Here's how the part is built. I have some questions about the finished solid (model axes, mm). A direction names the side the tool comes from. Coordinates: 2 decimals unless noted, no trailing zeros. Write each loop counter-clockwise with the first axis right and the second up, starting at its lowest first coordinate (ties: lowest second). Pieces come first, ordered by that corner, then holes. Notation, with made-up numbers: (30.25, 77.25) -> (87.25, 77.25) arc R12 cw to (87.25, 95.25) -> close; hole circle Ø2 at (44, 85.5). An arc over 180 degrees is marked (long way). Use a Markdown table: item, result. Add a question column.
Item 1: Imagine slicing it at B-B, the plane y = -6. Write out the boundary of the cut face in (x, z).
Item 2: If we mould it in two halves opening along X, with no side actions, what happens to faces 1 (the cylindrical face through (29.9, -19.94, 3.46)), 2 (the conical face through (-38.037, -20.598, 4.386)), 3 (the cylindrical face through (38.3, 20.74, 2.28))? For each: pulls with the +X half, pulls with the -X half, needs draft (parallel to the pull), parting line crosses it, or undercut.
Item 3: Will these pins go through, and if not, where does the flat tip stop? pin 1 Ø1.6 at (x, y) = (34, -18.5) entering from -Z; pin 2 Ø2.5 at (x, y) = (-35.3, 17.8) entering from -Z; pin 3 Ø1.5 at (x, y) = (23.5, 7) entering from +Z.
Item 4: On a 3-axis mill with a long thin cutter (end or side, diameter ignored), from which of +Z, -Z, +X, -X, +Y, -Y can I reach the whole of each face in a straight line? I mean faces 4 (the flat face through (37.67, -19.194, 1.331)), 5 (the conical face through (-38.098, 20.537, 4.386)), 6 (the flat face through (38.3, 4, 3)). Say none if no direction works.
Item 5: Imagine slicing it at A-A, the plane x = 0. Write out the boundary of the cut face in (y, z).
Item 6: If I drill on line 1 along X through (y, z) = (-17.8, 3.2); line 2 along X through (y, z) = (17.8, 3.15); line 3 along X through (y, z) = (9, 3.5), over which ranges is the centre line in solid material (lowest first)? Write a range as from..to.
Autodesk Fusion 360 part; units mm, degrees
sketch "Sketch1" plane through (0, 0, 0) normal (0, 0, 1) x (1, 0, 0)
  line L0 (39.5, 22) -> (-39.5, 22)
  line L1 (-39.5, 22) -> (-39.5, -22)
  line L2 (-39.5, -22) -> (39.5, -22)
  line L3 (39.5, -22) -> (39.5, 22)
  line L4 (39.5, 22) -> (-39.5, -22) construction
  line L5 (-39.5, 22) -> (39.5, -22) construction
  dimension "d1" = 44
  dimension "d2" = 79
extrude "Extrude1" add sketch "Sketch1" along normal blind 4.5
sketch "Sketch2" plane through (0, 0, 4.5) normal (0, 0, 1) x (-1, 0, 0)
  line L0 (-39.5, 22) -> (-39.5, -22)
  line L1 (-39.5, -22) -> (39.5, -22)
  line L2 (39.5, -22) -> (39.5, 22)
  line L3 (39.5, 22) -> (-39.5, 22)
  line L4 (-38.3, 20.8) -> (-38.3, -20.8)
  line L5 (-38.3, -20.8) -> (38.3, -20.8)
  line L6 (38.3, -20.8) -> (38.3, 20.8)
  line L7 (38.3, 20.8) -> (-38.3, 20.8)
  dimension "d5" = -1.2
extrude "Extrude2" cut sketch "Sketch2" against normal blind 2.1 contours L4 L5 L6 L7
sketch "Sketch3" plane through (0, 0, 2.4) normal (0, 0, 1) x (-1, 0, 0)
  line L0 (38.3, 20.8) -> (-38.3, 20.8)
  line L1 (-38.3, 20.8) -> (-38.3, -20.8)
  line L2 (-38.3, -20.8) -> (38.3, -20.8)
  line L3 (38.3, -20.8) -> (38.3, 20.8)
  line L4 (-38.3, -20.8) -> (-38.3, 20.8)
  line L5 (-38.3, 20.8) -> (38.3, 20.8)
  line L6 (38.3, 20.8) -> (38.3, -20.8)
  line L7 (38.3, -20.8) -> (-38.3, -20.8)
  line L8 (-39.5, 22) -> (-39.5, -22)
  line L9 (-39.5, -22) -> (39.5, -22)
  line L10 (39.5, -22) -> (39.5, 22)
  line L11 (39.5, 22) -> (-39.5, 22)
  circle A0 centre (35.3, -17.8) radius 4.5
  circle A1 centre (-35.3, 17.8) radius 4.5
  circle A2 centre (35.3, 17.8) radius 4.5
  dimension "d8" = 9
  dimension "d9" = 3
  dimension "d10" = 3
  dimension "d11" = 9
  dimension "d12" = 9
  dimension "d13" = 3
  dimension "d14" = 3
  dimension "d15" = 3
  dimension "d16" = 3
extrude "Extrude3" add sketch "Sketch3" along normal blind 2.1 contours L2 L3 L6 L7 A0
extrude "Extrude4" add sketch "Sketch3" along normal blind 2.1 contours L0 L3 L5 L6 A2
extrude "Extrude5" add sketch "Sketch3" along normal blind 2.1 contours L0 L1 L4 L5 A1
sketch "Sketch5" plane through (0, 0, 4.5) normal (0, 0, 1) x (-1, 0, 0)
  line L0 (-38.3, -20.8) -> (-38.3, 14.4459)
  arc A0 (-38.3, 14.4459) -> (-31.9459, 20.8) centre (-35.3, 17.8) ccw
  line L1 (-31.9459, 20.8) -> (31.9459, 20.8)
  arc A1 (31.9459, 20.8) -> (38.3, 14.4459) centre (35.3, 17.8) ccw
  line L2 (38.3, 14.4459) -> (38.3, -14.4459)
  arc A2 (38.3, -14.4459) -> (31.9459, -20.8) centre (35.3, -17.8) ccw
  line L3 (31.9459, -20.8) -> (-38.3, -20.8)
  line L4 (-39.5, 22) -> (-39.5, -22)
  line L5 (-39.5, -22) -> (39.5, -22)
  line L6 (39.5, -22) -> (39.5, 22)
  line L7 (39.5, 22) -> (-39.5, 22)
  circle A3 centre (35.3, -17.8) radius 1.65
  circle A4 centre (35.3, 17.8) radius 1.65
  circle A5 centre (-35.3, 17.8) radius 1.65
  point P0 (35.3, -17.8)
  dimension "d44" = 3.3
  dimension "d45" = 3.3
  dimension "d46" = 3.3
extrude "Extrude7" cut sketch "Sketch5" against normal blind 13 contours A3
extrude "Extrude8" cut sketch "Sketch5" against normal blind 18 contours A4
extrude "Extrude9" cut sketch "Sketch5" against normal blind 16 contours A5
sketch "Sketch6" plane through (0, 0, 0) normal (0, 0, 1) x (1, 0, 0)
  circle A0 centre (35.3, -17.8) radius 1.65
  circle A1 centre (-35.3, -17.8) radius 1.65
  circle A2 centre (-35.3, 17.8) radius 1.65
  line L0 (39.5, 22) -> (39.5, -22)
  line L1 (39.5, -22) -> (-39.5, -22)
  line L2 (-39.5, -22) -> (-39.5, 22)
  line L3 (-39.5, 22) -> (39.5, 22)
  line L4 (-32.1246, -17.8) -> (-33.7123, -15.05)
  line L5 (-33.7123, -15.05) -> (-36.8877, -15.05)
  line L6 (-36.8877, -15.05) -> (-38.4754, -17.8)
  line L7 (-38.4754, -17.8) -> (-36.8877, -20.55)
  line L8 (-36.8877, -20.55) -> (-33.7123, -20.55)
  line L9 (-33.7123, -20.55) -> (-32.1246, -17.8)
  line L10 (-32.1246, 17.8) -> (-33.7123, 20.55)
  line L11 (-33.7123, 20.55) -> (-36.8877, 20.55)
  line L12 (-36.8877, 20.55) -> (-38.4754, 17.8)
  line L13 (-38.4754, 17.8) -> (-36.8877, 15.05)
  line L14 (-36.8877, 15.05) -> (-33.7123, 15.05)
  line L15 (-33.7123, 15.05) -> (-32.1246, 17.8)
  line L16 (32.1246, -17.8) -> (33.7123, -20.55)
  line L17 (33.7123, -20.55) -> (36.8877, -20.55)
  line L18 (36.8877, -20.55) -> (38.4754, -17.8)
  line L19 (38.4754, -17.8) -> (36.8877, -15.05)
  line L20 (36.8877, -15.05) -> (33.7123, -15.05)
  line L21 (33.7123, -15.05) -> (32.1246, -17.8)
  point P0 (-35.3, -17.8)
  point P1 (-35.3, 17.8)
  point P2 (35.3, -17.8)
  dimension "d53" = 2.75
  dimension "d54" = 2.75
  dimension "d55" = 2.75
extrude "Extrude10" cut sketch "Sketch6" along normal blind 2.7 contours L10 L11 L12 L13 L14 L15
extrude "Extrude11" cut sketch "Sketch6" along normal blind 2.7 contours L16 L17 L18 L19 L20 L21
extrude "Extrude12" cut sketch "Sketch6" along normal blind 2.7 contours L4 L5 L6 L7 L8 L9
sketch "Sketch7" plane through (0, 0, 0) normal (0, 0, 1) x (1, 0, 0)
  line L0 (-36.8877, -20.55) -> (-33.7123, -20.55)
  line L1 (-33.7123, -20.55) -> (-32.1246, -17.8)
  line L2 (-32.1246, -17.8) -> (-33.7123, -15.05)
  line L3 (-33.7123, -15.05) -> (-36.8877, -15.05)
  line L4 (-36.8877, -15.05) -> (-38.4754, -17.8)
  line L5 (-38.4754, -17.8) -> (-36.8877, -20.55)
  line L6 (36.8877, -15.05) -> (33.7123, -15.05)
  line L7 (33.7123, -15.05) -> (32.1246, -17.8)
  line L8 (32.1246, -17.8) -> (33.7123, -20.55)
  line L9 (33.7123, -20.55) -> (36.8877, -20.55)
  line L10 (36.8877, -20.55) -> (38.4754, -17.8)
  line L11 (38.4754, -17.8) -> (36.8877, -15.05)
  line L12 (-36.8877, 15.05) -> (-33.7123, 15.05)
  line L13 (-33.7123, 15.05) -> (-32.1246, 17.8)
  line L14 (-32.1246, 17.8) -> (-33.7123, 20.55)
  line L15 (-33.7123, 20.55) -> (-36.8877, 20.55)
  line L16 (-36.8877, 20.55) -> (-38.4754, 17.8)
  line L17 (-38.4754, 17.8) -> (-36.8877, 15.05)
  line L18 (39.5, 22) -> (39.5, -22)
  line L19 (39.5, -22) -> (-39.5, -22)
  line L20 (-39.5, -22) -> (-39.5, 22)
  line L21 (-39.5, 22) -> (39.5, 22)
fillet "Fillet1" radius 3 2 edges at (-31.9459, 20.8, 3.45) (-38.3, 14.4459, 3.45)
fillet "Fillet2" radius 3 2 edges at (-31.9459, -20.8, 3.45) (-38.3, -14.4459, 3.45)
fillet "Fillet3" radius 3 2 edges at (31.9459, -20.8, 3.45) (38.3, -14.4459, 3.45)
fillet "Fillet4" radius 4.2 1 edges at (39.5, -22, 2.25)
fillet "Fillet5" radius 3 1 edges at (38.3, 20.8, 3.45)
fillet "Fillet6" radius 4.2 1 edges at (-39.5, -22, 2.25)
fillet "Fillet7" radius 4.2 1 edges at (-39.5, 22, 2.25)
fillet "Fillet8" radius 4.2 1 edges at (39.5, 22, 2.25)
chamfer "Chamfer1" distance 0.4 angle 45 8 edges at (0, -22, 4.5) (38.2698, -20.7698, 4.5) (39.5, 0, 4.5) (38.2698, 20.7698, 4.5) (0, 22, 4.5) (-38.2698, 20.7698, 4.5) (-39.5, 0, 4.5) (-38.2698, -20.7698, 4.5)
chamfer "Chamfer2" distance 0.4 angle 45 8 edges at (0, -22, 0) (38.2698, -20.7698, 0) (39.5, 0, 0) (38.2698, 20.7698, 0) (0, 22, 0) (-38.2698, 20.7698, 0) (-39.5, 0, 0) (-38.2698, -20.7698, 0)
equation "d53 = ( 5.5 / 2 ) * 1 mm"
equation "d54 = ( 5.5 / 2 ) * 1 mm"
equation "d55 = ( 5.5 / 2 ) * 1 mm"
Ans:
| question | item | result |
|---|---|---|
| 1 | outline | (-39.5, 0.4) -> (-39.1, 0) -> (39.1, 0) -> (39.5, 0.4) -> (39.5, 4.1) -> (39.1, 4.5) -> (38.3, 4.5) -> (38.3, 2.4) -> (-38.3, 2.4) -> (-38.3, 4.5) -> (-39.1, 4.5) -> (-39.5, 4.1) -> close |
| 2 | face 1 | undercut |
| 2 | face 2 | pulls with the -X half |
| 2 | face 3 | pulls with the +X half |
| 3 | pin 1 | stops at z = 2.7 |
| 3 | pin 2 | passes through |
| 3 | pin 3 | stops at z = 2.4 |
| 4 | face 4 | -Z |
| 4 | face 5 | +Z, -X, +Y |
| 4 | face 6 | +Z |
| 5 | outline | (-22, 0.4) -> (-21.6, 0) -> (21.6, 0) -> (22, 0.4) -> (22, 4.1) -> (21.6, 4.5) -> (20.8, 4.5) -> (20.8, 2.4) -> (-20.8, 2.4) -> (-20.8, 4.5) -> (-21.6, 4.5) -> (-22, 4.1) -> close |
| 6 | line 1 | x = -39.5..-36.95, -33.65..-30.8, 30.8..33.65, 36.95..39.5 |
| 6 | line 2 | x = -39.5..-36.95, -33.65..-30.8, 38.3..39.5 |
| 6 | line 3 | x = -39.5..-38.3, 38.3..39.5 |
